Part model, mm, in its own coordinate system. A direction names the side the tool comes from. Round coordinates to 2 decimals unless told otherwise and drop trailing zeros. Loops run counter-clockwise (first coordinate to the right, second up) from the corner with the lowest first, then second, coordinate; pieces in that order, holes last. Notation, with made-up numbers: (18.25, -34.5) -> (30.25, -34.5) arc R6 ccw to (30.25, -30.5) -> close; hole circle Ø7 at (22, -1.5). An arc over 180 degrees is marked (long way). Answer as CSV lines item,"result".
from build123d import *

# Parameters (mm, degrees)
CYLINDER341_R             = 1.25
CYLINDER341_DEPTH         = 10
CYLINDER342_R             = 1.25
CYLINDER342_DEPTH         = 10
CYLINDER343_R             = 1.25
CYLINDER343_DEPTH         = 10
CYLINDER344_R             = 1.25
CYLINDER344_DEPTH         = 10
CYLINDER346_R             = 1.25
CYLINDER346_DEPTH         = 10
CYLINDER345_R             = 1.25
CYLINDER345_DEPTH         = 10
CYLINDER339_R             = 1.25
CYLINDER339_DEPTH         = 10
CYLINDER340_R             = 1.25
CYLINDER340_DEPTH         = 10
BOX234_W                  = 10
BOX234_H                  = 10
BOX234_DEPTH              = 10
CYLINDER335_R             = 1.6
CYLINDER335_DEPTH         = 10
CYLINDER336_R             = 1.6
CYLINDER336_DEPTH         = 10
FUSION285_PLACEMENT_ANGLE = 120
CYLINDER338_R             = 1.6
CYLINDER338_DEPTH         = 10
CYLINDER337_R             = 1.6
CYLINDER337_DEPTH         = 10
CYLINDER333_R             = 1.6
CYLINDER333_DEPTH         = 10
CYLINDER334_R             = 1.6
CYLINDER334_DEPTH         = 10
FUSION284_PLACEMENT_ANGLE = 60
FUSION287_PLACEMENT_ANGLE = 30
CUT242_PLACEMENT_ANGLE    = 90
CYLINDER332_R             = 18.7
CYLINDER332_DEPTH         = 75
CYLINDER331_R             = 7
CYLINDER331_DEPTH         = 10
CYLINDER330_R             = 20.5
CYLINDER330_DEPTH         = 34
BOX233_W                  = 34
BOX233_H                  = 60
BOX233_DEPTH              = 17


with BuildPart() as cylinder341:
    # Cylinder341 → Cylinder341 (new body)
    with BuildSketch(Plane(origin=(87.5, 61, 14), x_dir=(1, 0, 0), z_dir=(0, -1, 0))):
        Circle(CYLINDER341_R)
    extrude(amount=CYLINDER341_DEPTH)


with BuildPart() as cylinder342:
    # Cylinder342 → Cylinder342 (new body)
    with BuildSketch(Plane(origin=(87.5, 11, 14), x_dir=(1, 0, 0), z_dir=(0, -1, 0))):
        Circle(CYLINDER342_R)
    extrude(amount=CYLINDER342_DEPTH)


with BuildPart() as fusion295:
    # Fusion295 base: copy of Cylinder342
    add(cylinder342.part)

    # Fusion295: union Cylinder341
    add(cylinder341.part)


with BuildPart() as fusion295_1:
    # Fusion295 placement: moved
    add(fusion295.part.moved(Location((251.5, 0, 0))))


with BuildPart() as cylinder343:
    # Cylinder343 → Cylinder343 (new body)
    with BuildSketch(Plane(origin=(87.5, 61, 14), x_dir=(1, 0, 0), z_dir=(0, -1, 0))):
        Circle(CYLINDER343_R)
    extrude(amount=CYLINDER343_DEPTH)


with BuildPart() as cylinder344:
    # Cylinder344 → Cylinder344 (new body)
    with BuildSketch(Plane(origin=(87.5, 11, 14), x_dir=(1, 0, 0), z_dir=(0, -1, 0))):
        Circle(CYLINDER344_R)
    extrude(amount=CYLINDER344_DEPTH)


with BuildPart() as fusion296:
    # Fusion296 base: copy of Cylinder344
    add(cylinder344.part)

    # Fusion296: union Cylinder343
    add(cylinder343.part)


with BuildPart() as fusion296_1:
    # Fusion296 placement: moved
    add(fusion296.part.moved(Location((261.5, 0, 0))))


with BuildPart() as cylinder346:
    # Cylinder346 → Cylinder346 (new body)
    with BuildSketch(Plane(origin=(87.5, 61, 14), x_dir=(1, 0, 0), z_dir=(0, -1, 0))):
        Circle(CYLINDER346_R)
    extrude(amount=CYLINDER346_DEPTH)


with BuildPart() as cylinder345:
    # Cylinder345 → Cylinder345 (new body)
    with BuildSketch(Plane(origin=(87.5, 11, 14), x_dir=(1, 0, 0), z_dir=(0, -1, 0))):
        Circle(CYLINDER345_R)
    extrude(amount=CYLINDER345_DEPTH)


with BuildPart() as fusion294:
    # Fusion294 base: copy of Cylinder345
    add(cylinder345.part)

    # Fusion294: union Cylinder346
    add(cylinder346.part)


with BuildPart() as fusion294_1:
    # Fusion294 placement: moved
    add(fusion294.part.moved(Location((270.5, 0, 0))))


with BuildPart() as cylinder339:
    # Cylinder339 → Cylinder339 (new body)
    with BuildSketch(Plane(origin=(87.5, 61, 14), x_dir=(1, 0, 0), z_dir=(0, -1, 0))):
        Circle(CYLINDER339_R)
    extrude(amount=CYLINDER339_DEPTH)


with BuildPart() as cylinder340:
    # Cylinder340 → Cylinder340 (new body)
    with BuildSketch(Plane(origin=(87.5, 11, 14), x_dir=(1, 0, 0), z_dir=(0, -1, 0))):
        Circle(CYLINDER340_R)
    extrude(amount=CYLINDER340_DEPTH)


with BuildPart() as fusion293:
    # Fusion297 base: copy of Cylinder340
    add(cylinder340.part)

    # Fusion297: union Cylinder339
    add(cylinder339.part)


with BuildPart() as fusion293_1:
    # Fusion297 placement: moved
    add(fusion293.part.moved(Location((242.5, 0, 0))))

    # Fusion293: union Fusion295, Fusion296, Fusion294
    add(fusion295_1.part)
    add(fusion296_1.part)
    add(fusion294_1.part)


with BuildPart() as fusion293_2:
    # Fusion293 placement: moved
    add(fusion293_1.part.moved(Location((0, 0, -8))))


with BuildPart() as fusion289:
    # Fusion289 base: copy of Cylinder342
    add(cylinder342.part)

    # Fusion289: union Cylinder341
    add(cylinder341.part)


with BuildPart() as fusion289_1:
    # Fusion289 placement: moved
    add(fusion289.part.moved(Location((251.5, 0, 0))))


with BuildPart() as fusion290:
    # Fusion290 base: copy of Cylinder344
    add(cylinder344.part)

    # Fusion290: union Cylinder343
    add(cylinder343.part)


with BuildPart() as fusion290_1:
    # Fusion290 placement: moved
    add(fusion290.part.moved(Location((261.5, 0, 0))))


with BuildPart() as fusion291:
    # Fusion291 base: copy of Cylinder345
    add(cylinder345.part)

    # Fusion291: union Cylinder346
    add(cylinder346.part)


with BuildPart() as fusion291_1:
    # Fusion291 placement: moved
    add(fusion291.part.moved(Location((270.5, 0, 0))))


with BuildPart() as fusion298:
    # Fusion288 base: copy of Cylinder340
    add(cylinder340.part)

    # Fusion288: union Cylinder339
    add(cylinder339.part)


with BuildPart() as fusion298_1:
    # Fusion288 placement: moved
    add(fusion298.part.moved(Location((242.5, 0, 0))))

    # Fusion292: union Fusion289, Fusion290, Fusion291
    add(fusion289_1.part)
    add(fusion290_1.part)
    add(fusion291_1.part)

    # Fusion298: union Fusion293
    add(fusion293_2.part)


with BuildPart() as cube314:
    # Box234 → Box234 (new body)
    with BuildSketch(Plane.XY):
        with Locations((5, 5)):
            Rectangle(BOX234_W, BOX234_H)
    extrude(amount=BOX234_DEPTH)


with BuildPart() as cylinder335:
    # Cylinder335 → Cylinder335 (new body)
    with BuildSketch(Plane(origin=(15.5, 0, 0), x_dir=(1, 0, 0), z_dir=(0, 0, 1))):
        Circle(CYLINDER335_R)
    extrude(amount=CYLINDER335_DEPTH)


with BuildPart() as fusion285:
    # Cylinder336 → Cylinder336 (new body)
    with BuildSketch(Plane(origin=(-15.5, 0, 0), x_dir=(1, 0, 0), z_dir=(0, 0, 1))):
        Circle(CYLINDER336_R)
    extrude(amount=CYLINDER336_DEPTH)

    # Fusion285: union Cylinder335
    add(cylinder335.part)


with BuildPart() as fusion285_1:
    # Fusion285 placement: moved
    add(fusion285.part.rotate(Axis((0, 0, 0), (0, 0, 1)), FUSION285_PLACEMENT_ANGLE))


with BuildPart() as cylinder338:
    # Cylinder338 → Cylinder338 (new body)
    with BuildSketch(Plane(origin=(15.5, 0, 0), x_dir=(1, 0, 0), z_dir=(0, 0, 1))):
        Circle(CYLINDER338_R)
    extrude(amount=CYLINDER338_DEPTH)


with BuildPart() as fusion286:
    # Cylinder337 → Cylinder337 (new body)
    with BuildSketch(Plane(origin=(-15.5, 0, 0), x_dir=(1, 0, 0), z_dir=(0, 0, 1))):
        Circle(CYLINDER337_R)
    extrude(amount=CYLINDER337_DEPTH)

    # Fusion286: union Cylinder338
    add(cylinder338.part)


with BuildPart() as cylinder333:
    # Cylinder333 → Cylinder333 (new body)
    with BuildSketch(Plane(origin=(15.5, 0, 0), x_dir=(1, 0, 0), z_dir=(0, 0, 1))):
        Circle(CYLINDER333_R)
    extrude(amount=CYLINDER333_DEPTH)


with BuildPart() as holes002:
    # Cylinder334 → Cylinder334 (new body)
    with BuildSketch(Plane(origin=(-15.5, 0, 0), x_dir=(1, 0, 0), z_dir=(0, 0, 1))):
        Circle(CYLINDER334_R)
    extrude(amount=CYLINDER334_DEPTH)

    # Fusion284: union Cylinder333
    add(cylinder333.part)


with BuildPart() as holes002_1:
    # Fusion284 placement: moved
    add(holes002.part.rotate(Axis((0, 0, 0), (0, 0, 1)), FUSION284_PLACEMENT_ANGLE))

    # Fusion287: union Fusion285, Fusion286
    add(fusion285_1.part)
    add(fusion286.part)


with BuildPart() as holes002_2:
    # Fusion287 placement: moved
    add(holes002_1.part.rotate(Axis((0, 0, 0), (0, 0, 1)), FUSION287_PLACEMENT_ANGLE))

    # Cut242: cut Cube314
    add(cube314.part, mode=Mode.SUBTRACT)


with BuildPart() as holes002_3:
    # Cut242 placement: moved
    add(holes002_2.part.moved(Location((327, 31, 5))).rotate(Axis((327, 31, 5), (0, 1, 0)), CUT242_PLACEMENT_ANGLE))


with BuildPart() as cylinder332:
    # Cylinder332 → Cylinder332 (new body)
    with BuildSketch(Plane(origin=(336, 31, 5), x_dir=(0, 0, -1), z_dir=(1, 0, 0))):
        Circle(CYLINDER332_R)
    extrude(amount=CYLINDER332_DEPTH)


with BuildPart() as cylinder331:
    # Cylinder331 → Cylinder331 (new body)
    with BuildSketch(Plane(origin=(327, 31, 12), x_dir=(0, 0, -1), z_dir=(1, 0, 0))):
        Circle(CYLINDER331_R)
    extrude(amount=CYLINDER331_DEPTH)


with BuildPart() as cylinder330:
    # Cylinder330 → Cylinder330 (new body)
    with BuildSketch(Plane(origin=(326, 31, 4.5), x_dir=(0, 0, -1), z_dir=(1, 0, 0))):
        Circle(CYLINDER330_R)
    extrude(amount=CYLINDER330_DEPTH)


with BuildPart() as motor_support001:
    # Box233 → Box233 (new body)
    with BuildSketch(Plane(origin=(326, 1, 1.5), x_dir=(1, 0, 0), z_dir=(0, 0, 1))):
        with Locations((17, 30)):
            Rectangle(BOX233_W, BOX233_H)
    extrude(amount=BOX233_DEPTH)

    # Fusion283: union Cylinder330
    add(cylinder330.part)


with BuildPart() as motor_support001_1:
    # Fusion283 placement: moved
    add(motor_support001.part.moved(Location((1, 0, 0))))

    # Cut240: cut Cylinder331
    add(cylinder331.part, mode=Mode.SUBTRACT)

    # Cut241: cut Cylinder332
    add(cylinder332.part, mode=Mode.SUBTRACT)

    # Cut243: cut holes002
    add(holes002_3.part, mode=Mode.SUBTRACT)

    # Cut244: cut Fusion298
    add(fusion298_1.part, mode=Mode.SUBTRACT)


with BuildPart() as motor_support001_2:
    # Cut244 placement: moved
    add(motor_support001_1.part.moved(Location((86, 0, 0))))


solid = motor_support001_2.part
Q1. Drill centre lines: line 1 along Z through (x, y) = (416, 54); line 2 along Y through (x, z) = (419, 12); line 3 along X through (y, z) = (56, 13.5). Where is each one in solid material? Low to high.
Geometry results:
line 1,"1.5 to 4.75, 7.25 to 12.75, 15.25 to 18.5"
line 2,"1 to 24, 38 to 61"
line 3,"413 to 414.85, 417.15 to 423.85, 426.15 to 433.85, 436.15 to 442.85, 445.15 to 447"
Q2. Saw through at C-C, the plane y = 56. Give the number of separate pieces and of enclosed holes in the cut face, then the cut area to 3 significant figures.
Geometry results:
separate pieces,"1"
enclosed holes,"8"
area,"539 mm2"
Q3. Saw through at B-B, the plane x = 444. Write the cut outline in (y, z), then the cut area to 3 significant figures.
Geometry results:
outline,"(1, 1.5) -> (10.72, 1.5) arc R20.5 ccw to (51.28, 1.5) -> (61, 1.5) -> (61, 4.75) -> (51, 4.75) -> (51, 7.25) -> (61, 7.25) -> (61, 12.75) -> (51, 12.75) -> (51, 15.25) -> (61, 15.25) -> (61, 18.5) -> (45.97, 18.5) arc R20.5 ccw to (16.03, 18.5) -> (1, 18.5) -> (1, 15.25) -> (11, 15.25) -> (11, 12.75) -> (1, 12.75) -> (1, 7.25) -> (11, 7.25) -> (11, 4.75) -> (1, 4.75) -> close; hole circle Ø37.4 at (31, 5)"
area,"494 mm2"
Q4. Which spindle directions (+Z, -Z, +X, -X, +Y, -Y) get a long thin tool onto all of the face, cutting with end or side? Do faces 5 (the face through (415.01, 6.07, 13.24)), 6 (the face through (417.44, 24.85, -8.49)), 7 (the face through (415.01, 56.07, 13.24)). Say none if no direction does.
Geometry results:
face 5,"-Y"
face 6,"+X, -X"
face 7,"+Y"
Q5. Two-plate mould, pull along Z, no slides. Class faces 1 (the face through (430, 1, 10)), 2 (the face through (430, 9, 18.5)), 3 (the face through (430, 56, 1.5)), 4 (the face through (415.01, 56.07, 5.24)): pulls with the +Z half, pulls with the -Z half, needs draft (parallel to the pull), parting line crosses it, or undercut.
Geometry results:
face 1,"needs draft"
face 2,"pulls with the +Z half"
face 3,"pulls with the -Z half"
face 4,"undercut"
Q6. Drop flat-ended pins along their axis: P1, Ø0.8, axis at x = 435, z = 14.5, coming from the +Y side; P2, Ø12, axis at x = 420, y = 10, coming from the -Z side; P3, Ø3, axis at x = 425, y = 49.5, coming from the +Z side. Give the stop position or say it passes through.
Geometry results:
P1,"y = 51"
P2,"z = -9.47"
P3,"z = 18.5"
Q7. Saw through at A-A, the plane y = 31. Write the cut outline in (x, z), then the cut area to 3 significant figures.
Geometry results:
outline,"(413, -16) -> (447, -16) -> (447, -13.7) -> (422, -13.7) -> (422, 5) -> (413, 5) -> close; (413, 19) -> (422, 19) -> (422, 23.7) -> (447, 23.7) -> (447, 25) -> (413, 25) -> close"
area,"333 mm2"
